```python
from build123d import *

# Parameters (mm, degrees)
SCHIZZO1_R                     = 67.5
ESTRUSIONE_ESTRUSIONE1_DEPTH   = 5
SCHIZZO2_R                     = 45
ESTRUSIONE_ESTRUSIONE2_DEPTH   = 6
SCHIZZO3_R                     = 35
TAGLIO_ESTRUSIONE1_DEPTH       = 8
SCHIZZO4_R                     = 26
TAGLIO_ESTRUSIONE2_DEPTH       = 4
SMUSSO1_SIZE                   = 1
FORO_PER_VITE_M8_1_D           = 9
FORO_PER_VITE_M8_1_CSINK_D     = 9.05
FORO_PER_VITE_M8_1_CSINK_ANGLE = 90
RIPETIZIONECIRCOLARE1_COUNT    = 6
SCHIZZO8_R                     = 52.5
SCHIZZO8_R_2                   = 49.5
TAGLIO_ESTRUSIONE3_DEPTH       = 1.5


with BuildPart() as part:
    # Schizzo1 → Estrusione-Estrusione1 (new body)
    with BuildSketch(Plane.XY):
        Circle(SCHIZZO1_R)
    extrude(amount=ESTRUSIONE_ESTRUSIONE1_DEPTH)

    # Schizzo2 → Estrusione-Estrusione2 (add)
    with BuildSketch(Plane.XY.offset(5)):
        Circle(SCHIZZO2_R)
    extrude(amount=ESTRUSIONE_ESTRUSIONE2_DEPTH)

    # Schizzo3 → Taglio-Estrusione1 (cut)
    with BuildSketch(Plane.XY.offset(11)):
        Circle(SCHIZZO3_R)
    extrude(amount=-TAGLIO_ESTRUSIONE1_DEPTH, mode=Mode.SUBTRACT)

    # Schizzo4 → Taglio-Estrusione2 (cut, through all)
    with BuildSketch(Plane.XY.offset(3)):
        Circle(SCHIZZO4_R)
    extrude(amount=-TAGLIO_ESTRUSIONE2_DEPTH, mode=Mode.SUBTRACT)

    # Smusso1
    smusso1_edges = [part.edges().sort_by_distance(p)[0] for p in [
        (-67.5, 0, 0),
        (-45, 0, 11),
    ]]
    chamfer(smusso1_edges, length=SMUSSO1_SIZE)

    # Foro per Vite M8-1 (through all)
    with Locations(Plane(origin=(0, 0, 0), x_dir=(-1, 0, 0), z_dir=(0, 0, -1))):
        with Locations((0, 60)):
            foro_per_vite_m8_1 = CounterSinkHole(FORO_PER_VITE_M8_1_D / 2, FORO_PER_VITE_M8_1_CSINK_D / 2, counter_sink_angle=FORO_PER_VITE_M8_1_CSINK_ANGLE)

    # RipetizioneCircolare1: Foro per Vite M8-1 ×6 about axis
    ripetizionecircolare1_axis = Axis((0, 0, 0), (0, 0, 1))
    for i in range(1, RIPETIZIONECIRCOLARE1_COUNT):
        add(foro_per_vite_m8_1.rotate(ripetizionecircolare1_axis, i * 360 / RIPETIZIONECIRCOLARE1_COUNT), mode=Mode.SUBTRACT)

    # Schizzo8 → Taglio-Estrusione3 (cut)
    with BuildSketch(Plane.XY.offset(5)):
        Circle(SCHIZZO8_R)
        Circle(SCHIZZO8_R_2, mode=Mode.SUBTRACT)
    extrude(amount=-TAGLIO_ESTRUSIONE3_DEPTH, mode=Mode.SUBTRACT)


solid = part.part
```
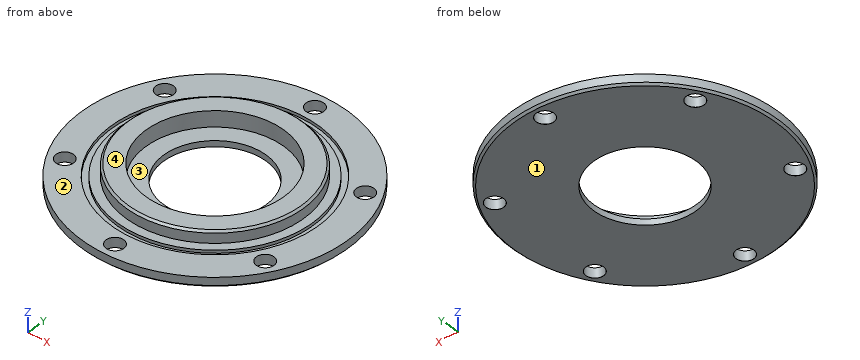
Model file for the job. Use its own axes, mm. Face numbers are marked on the shaded views. A direction names the side the tool comes from. Coordinates: 2 decimals unless noted, no trailing zeros. Write each loop counter-clockwise with the first axis right and the second up, starting at its lowest first coordinate (ties: lowest second). Pieces come first, ordered by that corner, then holes. Notation, with made-up numbers: (-33, 4) - (19, 4) arc R17 ccw to (19, 21) - close; hole circle Ø2 at (14, 75.5). An arc over 180 degrees is marked (long way). One line per item, written item: value. Start each with the question number.
1. Slice it at A-A (y = 0). Write the cut outline in (x, z), plus the area to 3 significant figures.
2. Mould opens along Y. For the marked faces 3 and 4 say: released by +Y, released by -Y, zero draft, split by the parting line, or undercut.
3. Slice it at C-C (x = 0). Count the separate pieces of the cut face and the enclosed holes in it, plus the area to 3 significant figures.
4. Tool access for the marked faces 1 and 2: list every direction of +Z, -Z, +X, -X, +Y, -Y with a clear straight run to the whole face (end or side of a thin tool).
5. Probe line 1 (Y direction, x = 0, z = 2.25); line 2 (Y direction, x = 0, z = 4.5); line 3 (X direction, y = -30, z = 1.2). List the from-to ranges inside material, lowest first. Write a range as from..to.
6. Slice it at B-B (z = 8.25). Write the cut outline in (x, y).
7. Flat gauge pins, fed straight in: pin 1 (2 mm diameter, centred on x = 26, y = -41.5, fed in from +Z); pin 2 (6 mm diameter, centred on y = 44.5, z = 2, fed in from -X); pin 3 (5 mm diameter, centred on y = 5, z = 6.5, fed in from +X). Where does each tip first touch, or does it go through?
Answers below:
1. outline: (-67.5, 1) - (-66.5, 0) - (-26, 0) - (-26, 3) - (-35, 3) - (-35, 11) - (-44, 11) - (-45, 10) - (-45, 5) - (-49.5, 5) - (-49.5, 3.5) - (-52.5, 3.5) - (-52.5, 5) - (-67.5, 5) - close; (26, 0) - (66.5, 0) - (67.5, 1) - (67.5, 5) - (52.5, 5) - (52.5, 3.5) - (49.5, 3.5) - (49.5, 5) - (45, 5) - (45, 10) - (44, 11) - (35, 11) - (35, 3) - (26, 3) - close
1. area: 488 mm^2
2. face 3: undercut
2. face 4: zero draft
3. separate pieces: 4
3. enclosed holes: 0
3. area: 398 mm^2
4. face 1: -Z, +X, -X, +Y, -Y
4. face 2: +Z
5. line 1: y = -67.5..-64.5, -55.5..-26, 26..55.5, 64.5..67.5
5. line 2: y = -67.5..-64.5, -55.5..-52.5, -49.5..-35, 35..49.5, 52.5..55.5, 64.5..67.5
5. line 3: x = -60.47..-56.46, -47.46..47.46, 56.46..60.47
6. outline: circle Ø90 at (0, 0); hole circle Ø70 at (0, 0)
7. pin 1: stops at z = 5
7. pin 2: stops at x = -53.24
7. pin 3: stops at x = 67.43
